Read the model definition and answer for the solid it produces. Units are mm, in the model's axes. Face numbers are marked on the shaded views. A direction names the side the tool comes from. Give positions to 0.01 mm unless a question says otherwise; leave off trailing zeros. Write each loop counter-clockwise with the first axis right and the second up, starting at its lowest first coordinate (ties: lowest second). Pieces come first, ordered by that corner, then holes. Notation, with made-up numbers: (-16.75, 14.5) -> (36.25, 14.5) arc R12 ccw to (36.25, 25.5) -> close; hole circle Ø6 at (77.5, 71). An arc over 180 degrees is marked (long way). Put each result on its own line as item: value. Start each with the question number.
Autodesk Fusion 360 part; units mm, degrees
sketch "Sketch1" plane through (0, 0, 0) normal (0, 1, 0) x (1, 0, 0)
  line L0 (26.45, 12.95) -> (-26.45, 12.95)
  line L1 (-26.45, 12.95) -> (-26.45, -12.95)
  line L2 (-26.45, -12.95) -> (26.45, -12.95)
  line L3 (26.45, -12.95) -> (26.45, 12.95)
  line L4 (26.45, 12.95) -> (-26.45, -12.95) construction
  line L5 (-26.45, 12.95) -> (26.45, -12.95) construction
  line L6 (26.45, -15.45) -> (-26.45, -15.45)
  line L7 (-26.45, -15.45) -> (-26.45, 15.45)
  line L8 (-26.45, 15.45) -> (26.45, 15.45)
  line L9 (26.45, 15.45) -> (26.45, -15.45)
  line L10 (26.45, -15.45) -> (-26.45, 15.45) construction
  line L11 (-26.45, -15.45) -> (26.45, 15.45) construction
  dimension "d1" = 52.9
  dimension "d2" = 25.9
  dimension "d9" = 2.5
extrude "Extrude1" add sketch "Sketch1" along normal blind 2 contours L0 L1 L2 L3 L7 L9
sketch "Sketch2" plane through (0, 2, 0) normal (0, 1, 0) x (-1, 0, 0)
  line L0 (-26.45, 12.95) -> (-26.45, -12.95)
  line L1 (-26.45, -12.95) -> (26.45, -12.95)
  line L2 (26.45, -12.95) -> (26.45, 12.95)
  line L3 (26.45, 12.95) -> (-26.45, 12.95)
  line L4 (21.45, -2.5) -> (31.45, -2.5)
  line L5 (31.45, -2.5) -> (31.45, 2.5)
  line L6 (31.45, 2.5) -> (21.45, 2.5)
  line L7 (21.45, 2.5) -> (21.45, -2.5)
  line L8 (21.45, -2.5) -> (31.45, 2.5) construction
  line L9 (31.45, -2.5) -> (21.45, 2.5) construction
  point P0 (26.45, 0)
  dimension "d5" = 10
  dimension "d6" = 5
extrude "Extrude2" add sketch "Sketch2" along normal mid plane 2 contours L2 L4 L5 L6 | L2 L4 L6 L7
extrude "Extrude3" add sketch "Sketch1" along normal blind 0.5
sketch "Sketch3" plane through (0, 0, 0) normal (0, 0, 1) x (1, 0, 0)
  line L0 (26.45, 0.5) -> (-26.45, 0.5)
  line L1 (-26.45, 0.5) -> (-26.45, 2)
  line L2 (-26.45, 2) -> (26.45, 2)
  line L3 (26.45, 2) -> (26.45, 0.5)
  line L4 (26.45, 0) -> (-26.45, 0)
  line L5 (-26.45, 0) -> (-26.45, 0.5)
  line L6 (-26.45, 0.5) -> (26.45, 0.5)
  line L7 (26.45, 0.5) -> (26.45, 0)
  line L8 (26.45, 0) -> (28.55, 0)
  line L9 (28.55, 0) -> (28.55, 2)
  line L10 (28.55, 2) -> (26.45, 2)
  line L11 (26.45, 2) -> (26.45, 0)
  line L12 (28.55, 0) -> (29.55, 0)
  line L13 (29.55, 0) -> (29.55, 5.95)
  line L14 (29.55, 5.95) -> (28.55, 5.95)
  line L15 (28.55, 5.95) -> (28.55, 0)
  line L16 (28.55, 5.95) -> (27.55, 5.95)
  line L17 (27.55, 5.95) -> (27.55, 4.05)
  line L18 (27.55, 4.05) -> (28.55, 4.05)
  line L19 (28.55, 4.05) -> (28.55, 5.95)
  line L20 (28.55, 5.95) -> (27.55, 4.05)
  line L21 (27.55, 5.95) -> (28.55, 4.05) construction
  line L22 (29.55, 5.95) -> (28.4726, 5.3162)
  line L23 (28.4726, 5.3162) -> (31.9726, -0.6338)
  line L24 (31.9726, -0.6338) -> (33.05, 0)
  line L25 (33.05, 0) -> (29.55, 5.95)
  line L26 (33.05, 0) -> (33.05, -1.5)
  line L27 (33.05, -1.5) -> (31.9726, -1.5)
  line L28 (31.9726, -1.5) -> (31.9726, -0.6338)
  line L29 (33.05, 0) -> (29.55, 0) construction
  point P0 (28.05, 5)
  dimension "d12" = 2.1
  dimension "d13" = 2
  dimension "d14" = 1
  dimension "d17" = 3
  dimension "d18" = 1.9
  dimension "d19" = 1
  dimension "d20" = 1.25
  dimension "d21" = 3.5
  dimension "d27" = 1.5
sketch "Sketch4" plane through (0, 0, 0) normal (0, 0, 1) x (1, 0, 0)
  line L0 (26.45, 0.5) -> (-26.45, 0.5)
  line L1 (-26.45, 0.5) -> (-26.45, 2)
  line L2 (-26.45, 2) -> (26.45, 2)
  line L3 (26.45, 2) -> (26.45, 0.5)
  line L4 (26.45, 0) -> (-26.45, 0)
  line L5 (-26.45, 0) -> (-26.45, 0.5)
  line L6 (-26.45, 0.5) -> (26.45, 0.5)
  line L7 (26.45, 0.5) -> (26.45, 0)
  line L8 (28.55, 2) -> (26.45, 2)
  line L9 (26.45, 0) -> (28.55, 0)
  line L10 (28.55, 0) -> (29.55, 0)
  line L11 (29.55, 0) -> (29.55, 5.95)
  line L12 (28.55, 0) -> (28.55, 2)
  line L13 (26.45, 0) -> (33.25, 0)
  line L14 (33.25, 0) -> (33.25, 2.8)
  line L15 (33.25, 2.8) -> (26.45, 2.8)
  line L16 (26.45, 2.8) -> (26.45, 0)
  dimension "d30" = 6.8
  dimension "d34" = 2.8
extrude "Extrude6" add sketch "Sketch4" along normal mid plane 7.8 contours L3 L7 L8 L9 L12 L13 L16 | L8 L10 L11 L12 L13 L15 L16 | L11 L13 L14 L15
sketch "Sketch6" plane through (0, 2.8, 0) normal (0, 1, 0) x (-1, 0, 0)
  line L0 (-26.45, -3.9) -> (-26.45, 3.9)
  line L1 (-26.45, 3.9) -> (-33.25, 3.9)
  line L2 (-33.25, 3.9) -> (-33.25, -3.9)
  line L3 (-33.25, -3.9) -> (-26.45, -3.9)
  circle A0 centre (-30, -0.1) radius 2.05
  dimension "d35" = 4.1
  dimension "d38" = 4
  dimension "d39" = 3.55
extrude "Extrude8" cut sketch "Sketch6" against normal blind 2.5 contours A0
chamfer "Chamfer1" distance 0.4 angle 45 1 edges at (31.9113, 2.8, 0.6413)
chamfer "Chamfer2" distance 0.8 angle 45 1 edges at (26.45, 2, 0)
fillet "Fillet1" radius 1 2 edges at (33.25, 1.4, -3.9) (33.25, 1.4, 3.9)
fillet "Fillet2" radius 1.5 8 edges at (26.45, 1.25, 12.95) (26.45, 0.25, 15.45) (26.45, 1.25, -12.95) (26.45, 0.25, -15.45) (-26.45, 0.25, -15.45) (-26.45, 1.25, -12.95) (-26.45, 0.25, 15.45) (-26.45, 1.25, 12.95)
extrude "Extrude4" [suppressed]
extrude "Extrude5" [suppressed]
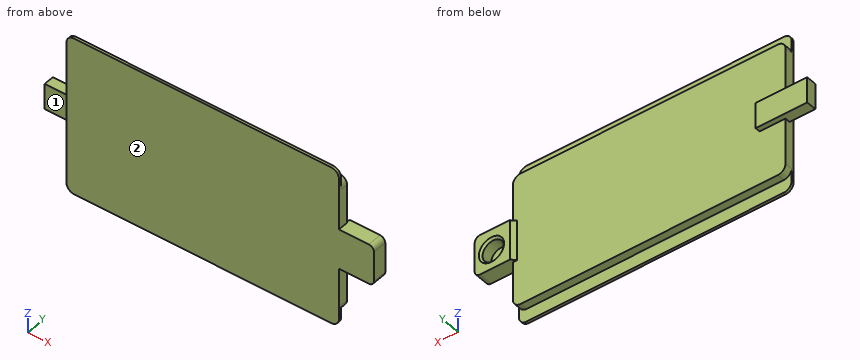
1) For the marked faces 1 and 2, determine the directions among +Z, -Z, +X, -X, +Y, -Y from which every point of the face is accessible in a straight line to the end or side of a thin tool.
2) A cutting plane is placed at D-D on z = 8. Give the vertices of the cut face in (x, y).
3) Each of these flat-tipped pins is pushed along its axis until it touches: pin 1 Ø1 at (x, y) = (-26.5, 2) entering from +Z; pin 2 Ø4.5 at (x, z) = (30, 0) entering from +Y; pin 3 Ø0.8 at (x, y) = (28, 1.5) entering from -Z. Where does it stop, or does it pass through?
4) A cutting plane is placed at C-C on x = 11. Give the vertices of the cut face in (y, z).
5) Straight lines are drawn through the part: line 1 (Z direction, x = 30, y = 1.5); line 2 (Z direction, x = -14, y = 1.5); line 3 (Y direction, x = -4.5, z = -2). For each, find the intervals that lie inside material, in ascending order. Write a range as [from, to].
6) A cutting plane is placed at A-A on x = 30. Give the vertices of the cut face in (y, z), and give its area (3 significant figures).
Results found:
1. face 1: +Z, -Z, -X, -Y
1. face 2: +Z, -Z, +X, -X, -Y
2. outline: (-26.45, 0) -> (26.45, 0) -> (26.45, 2) -> (-26.45, 2) -> close
3. pin 1: stops at z = 12.52
3. pin 2: stops at y = 2.7
3. pin 3: stops at z = -3.9
4. outline: (0, -15.45) -> (0.5, -15.45) -> (0.5, -12.95) -> (2, -12.95) -> (2, 12.95) -> (0.5, 12.95) -> (0.5, 15.45) -> (0, 15.45) -> close
5. line 1: z = [-3.9, -2.15], [1.95, 3.9]
5. line 2: z = [-12.95, 12.95]
5. line 3: y = [0, 2]
6. outline: (0, -3.9) -> (2.8, -3.9) -> (2.8, -2.55) -> (2.4, -2.15) -> (0.3, -2.15) -> (0.3, 1.95) -> (2.4, 1.95) -> (2.8, 2.35) -> (2.8, 3.9) -> (0, 3.9) -> close
6. area: 11.4 mm²
